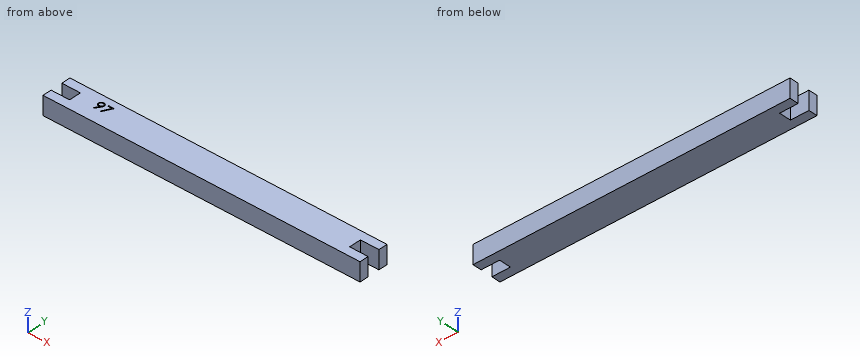
from build123d import *

# Parameters (mm, degrees)
BOSS_EXTRUDE1_DEPTH = 6.2
CUT_EXTRUDE1_DEPTH  = 1


with BuildPart() as part:
    # Sketch1 → Boss-Extrude1 (new body)
    with BuildSketch(Plane.XY):
        Polygon((0, 3), (-6.2, 3), (-6.2, 0), (100, 0), (100, 3), (93.8, 3), (93.8, 7), (100, 7), (100, 10), (-6.2, 10), (-6.2, 7), (0, 7), align=None)
    extrude(amount=BOSS_EXTRUDE1_DEPTH)

    # Sketch2 → Cut-Extrude1 (cut)
    with BuildSketch(Plane.XY.offset(6.2)):
        with BuildLine():
            Line((6.875309832, 4.402369049), (6.647615521, 4.560737438))
            Line((6.647615521, 4.560737438), (7.530407989, 5.851217206))
            add(Edge.make_bspline(
                [(7.530407989, 5.851217206), (7.474082821, 5.844329213), (7.363175427, 5.83076637), (7.251472484, 5.828274762), (7.196498734, 5.827048536)],
                knots=[0, 0, 0, 0, 0.000170115, 0.000334967, 0.000334967, 0.000334967, 0.000334967], degree=3))
            add(Edge.make_bspline(
                [(7.196498734, 5.827048536), (7.163168448, 5.827902227), (7.097744011, 5.829577947), (7.001558154, 5.842860159), (6.909133396, 5.863316346), (6.820714766, 5.893840574), (6.735969929, 5.931775664), (6.655083889, 5.978817383), (6.578165531, 6.034158805), (6.506040952, 6.097507304), (6.440443875, 6.167065252), (6.382002741, 6.240685014), (6.333433285, 6.319221787), (6.293086668, 6.401073486), (6.262488328, 6.487416569), (6.240206598, 6.577268525), (6.226488462, 6.671259086), (6.224856425, 6.735235454), (6.22402778, 6.767718608)],
                knots=[0, 0, 0, 0, 9.9954e-05, 0.000196201, 0.000290782, 0.000383503, 0.000476303, 0.000568919, 0.000663705, 0.000760153, 0.000856434, 0.000950205, 0.001041624, 0.001132931, 0.001223461, 0.001315861, 0.001410305, 0.001507717, 0.001507717, 0.001507717, 0.001507717], degree=3))
            add(Edge.make_bspline(
                [(6.22402778, 6.767718608), (6.225601161, 6.812140172), (6.228689387, 6.89933069), (6.253543756, 7.02672418), (6.294419921, 7.147180545), (6.351414234, 7.260383078), (6.423200731, 7.364703363), (6.509477809, 7.458691172), (6.609720691, 7.541009718), (6.721645809, 7.61177056), (6.842616049, 7.668680165), (6.969315474, 7.710625816), (7.100773283, 7.735298966), (7.189825384, 7.738551854), (7.234659792, 7.740189562)],
                knots=[0, 0, 0, 0, 0.000133185, 0.000261414, 0.000387724, 0.00051373, 0.000640399, 0.00076644, 0.000895188, 0.001028407, 0.001162697, 0.001295241, 0.001427846, 0.0015623, 0.0015623, 0.0015623, 0.0015623], degree=3))
            add(Edge.make_bspline(
                [(7.234659792, 7.740189562), (7.278645715, 7.738529342), (7.365557754, 7.735248905), (7.49336421, 7.711224162), (7.61577499, 7.670732323), (7.732111513, 7.614775612), (7.839825123, 7.544634503), (7.936686037, 7.461055328), (8.020483848, 7.363986028), (8.091081225, 7.255774326), (8.147750476, 7.139508565), (8.188637476, 7.018147435), (8.213806734, 6.892563738), (8.216978402, 6.807478751), (8.218579062, 6.76453852)],
                knots=[0, 0, 0, 0, 0.000131915, 0.000260652, 0.000388569, 0.000517718, 0.000646848, 0.000773094, 0.000900237, 0.001030248, 0.001159674, 0.001287189, 0.001413545, 0.001542287, 0.001542287, 0.001542287, 0.001542287], degree=3))
            add(Edge.make_bspline(
                [(8.218579062, 6.76453852), (8.217510077, 6.731206674), (8.215341908, 6.663601362), (8.200159687, 6.560885266), (8.174378519, 6.456154507), (8.14512162, 6.36750706), (8.116880297, 6.294292966), (8.090299985, 6.236461176), (8.060806817, 6.175590744), (8.02640908, 6.112319945), (7.989431853, 6.045842216), (7.947649509, 5.976824324), (7.902015169, 5.905173652), (7.869512495, 5.856870936), (7.852868926, 5.832136677)],
                knots=[0, 0, 0, 0, 9.9984e-05, 0.000202793, 0.000310776, 0.000423207, 0.000482616, 0.000546097, 0.000614079, 0.0006855, 0.000762103, 0.000842274, 0.000927493, 0.001016928, 0.001016928, 0.001016928, 0.001016928], degree=3))
            Line((7.852868926, 5.832136677), (6.875309832, 4.402369049))
        make_face()
        with BuildLine():
            add(Edge.make_bspline(
                [(7.249288197, 6.152689562), (7.274537624, 6.153379338), (7.323689675, 6.154722099), (7.395696225, 6.162894769), (7.463663181, 6.177385456), (7.5277721, 6.198176909), (7.588665789, 6.223265459), (7.64537703, 6.25520776), (7.697953284, 6.293322851), (7.746746618, 6.336149079), (7.790075389, 6.383729251), (7.828667995, 6.43352877), (7.861470796, 6.485766237), (7.887381769, 6.541095839), (7.908685633, 6.598170736), (7.923397687, 6.657910044), (7.931547761, 6.720002521), (7.932937118, 6.762183447), (7.933643165, 6.783619049)],
                knots=[0, 0, 0, 0, 7.5753e-05, 0.000147465, 0.000217073, 0.000283852, 0.000349411, 0.000414338, 0.000478589, 0.000543925, 0.000608743, 0.000671332, 0.000732749, 0.000793345, 0.000854313, 0.000915245, 0.00097749, 0.001041807, 0.001041807, 0.001041807, 0.001041807], degree=3))
            add(Edge.make_bspline(
                [(7.933643165, 6.783619049), (7.933035679, 6.805063602), (7.931838555, 6.847322725), (7.922234361, 6.909507132), (7.905338623, 6.969100305), (7.882668683, 7.026428495), (7.852805325, 7.081020689), (7.81697002, 7.133562287), (7.774395583, 7.183720146), (7.725407541, 7.230314617), (7.672580482, 7.273265925), (7.616282743, 7.311171866), (7.556978355, 7.342941094), (7.495029125, 7.369156588), (7.43030598, 7.38961427), (7.362847219, 7.404325737), (7.292311958, 7.4124644), (7.244431791, 7.413844975), (7.220031386, 7.414548536)],
                knots=[0, 0, 0, 0, 6.4316e-05, 0.000126743, 0.000188161, 0.000249812, 0.000311283, 0.000374438, 0.00044032, 0.000508243, 0.00057698, 0.000644365, 0.000711521, 0.0007785, 0.000845884, 0.000914871, 0.00098532, 0.001058531, 0.001058531, 0.001058531, 0.001058531], degree=3))
            add(Edge.make_bspline(
                [(7.220031386, 7.414548536), (7.19584319, 7.413843839), (7.148386148, 7.412461228), (7.078477946, 7.404341207), (7.011475315, 7.389515332), (6.946939703, 7.369166064), (6.884992313, 7.342939138), (6.825690722, 7.311170201), (6.769379814, 7.273274651), (6.716603403, 7.230280821), (6.66752886, 7.183937028), (6.625686416, 7.133342561), (6.589769099, 7.08104802), (6.559946775, 7.026421231), (6.53726592, 6.969102243), (6.520373105, 6.909506607), (6.510768126, 6.847322862), (6.509571109, 6.805063648), (6.508963678, 6.783619049)],
                knots=[0, 0, 0, 0, 7.2576e-05, 0.000142393, 0.000210758, 0.000278143, 0.000345121, 0.000412278, 0.000479663, 0.0005484, 0.000616323, 0.000681795, 0.00074495, 0.000806421, 0.000868072, 0.00092949, 0.000991917, 0.001056233, 0.001056233, 0.001056233, 0.001056233], degree=3))
            add(Edge.make_bspline(
                [(6.508963678, 6.783619049), (6.509513339, 6.762166754), (6.510597373, 6.719858903), (6.521054725, 6.657695675), (6.538542879, 6.598107099), (6.561964754, 6.540513772), (6.592809054, 6.48547573), (6.630658545, 6.433253908), (6.675022861, 6.383256321), (6.725308954, 6.336259779), (6.780343643, 6.293123163), (6.839123548, 6.255449173), (6.900636757, 6.223633456), (6.965099808, 6.198105201), (7.032034976, 6.177593192), (7.102043846, 6.162921475), (7.17489489, 6.154800491), (7.224252516, 6.153399956), (7.249288197, 6.152689562)],
                knots=[0, 0, 0, 0, 6.4316e-05, 0.000126844, 0.000188436, 0.000250326, 0.000312966, 0.000377217, 0.000443451, 0.000513196, 0.000583426, 0.000652939, 0.000722346, 0.000790847, 0.000860662, 0.000932137, 0.001005113, 0.00108023, 0.00108023, 0.00108023, 0.00108023], degree=3))
        make_face(mode=Mode.SUBTRACT)
        Polygon((8.829155986, 7.658779305), (10.783002139, 7.658779305), (9.114091883, 4.402369049), (8.867953061, 4.537840804), (10.300900777, 7.33313828), (8.829155986, 7.33313828), align=None)
    extrude(amount=-CUT_EXTRUDE1_DEPTH, mode=Mode.SUBTRACT)


solid = part.part
CAD build for the part. Positions are in the model's coordinates, mm. Round coordinates to 2 decimals unless told otherwise and drop trailing zeros. Loops run counter-clockwise (first coordinate to the right, second up) from the corner with the lowest first, then second, coordinate; pieces in that order, holes last.
(1) Drop flat-ended pins along their axis: pin 1 (3 mm diameter, centred on x = 98.5, z = 4.5, fed in from -Y); pin 2 (1.2 mm diameter, centred on y = 6, z = 3.5, fed in from -X); pin 3 (2 mm diameter, centred on y = 5.5, z = 3.5, fed in from +X). Give the stop position or say it passes through.
(2) Wall check: line 1 along X through (y, z) = (5, 5); line 2 along Y through (x, z) = (94.5, 3.5). Give the ranges that are in metal, low to high.
(3) Cut at A-A (z = 3). Give the cut face in (x, y).
Findings below:
1. pin 1: stops at y = 0
1. pin 2: stops at x = 0
1. pin 3: stops at x = 93.8
2. line 1: x = 0 to 93.8
2. line 2: y = 0 to 3, 7 to 10
3. outline: (-6.2, 0) - (100, 0) - (100, 3) - (93.8, 3) - (93.8, 7) - (100, 7) - (100, 10) - (-6.2, 10) - (-6.2, 7) - (0, 7) - (0, 3) - (-6.2, 3) - close
